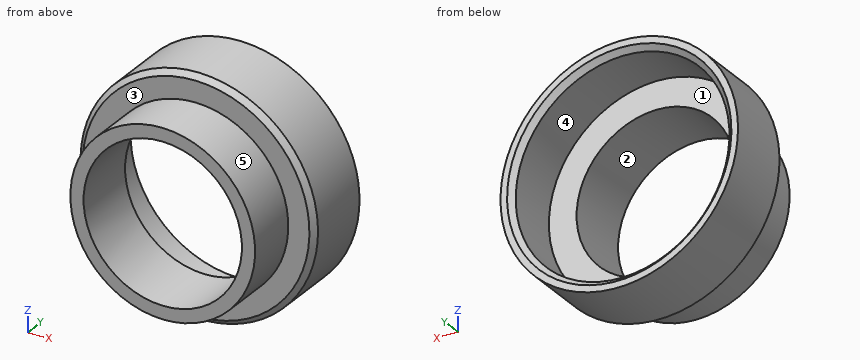
from build123d import *

# Parameters (mm, degrees)
SCHIZZO1_R        = 35
SCHIZZO1_R_2      = 30
ESTRUSIONE1_DEPTH = 30
ESTRUSIONE2_START = -10
SCHIZZO2_R        = 45
SCHIZZO2_R_2      = 30
ESTRUSIONE2_DEPTH = 5
SCHIZZO3_R        = 45
SCHIZZO3_R_2      = 40.5
ESTRUSIONE3_DEPTH = 22
SMUSSO1_SIZE      = 2
SMUSSO2_SIZE      = 2
SCHIZZO4_R        = 40.5
ESTRUSIONE4_DEPTH = 20


with BuildPart() as part:
    # Schizzo1 → Estrusione1 (new body)
    with BuildSketch(Plane(origin=(0, 0, 0), x_dir=(1, 0, 0), z_dir=(0, 1, 0))):
        with Locations(Location((0, 0, 0), (0, 0, 270))):
            Circle(SCHIZZO1_R)
        with Locations(Location((0, 0, 0), (0, 0, 270))):
            Circle(SCHIZZO1_R_2, mode=Mode.SUBTRACT)
    extrude(amount=ESTRUSIONE1_DEPTH)

    # Schizzo2 → Estrusione2 (add)
    with BuildSketch(Plane(origin=(0, 30, 0), x_dir=(1, 0, 0), z_dir=(0, 1, 0)).offset(ESTRUSIONE2_START)):
        with Locations(Location((0, 0, 0), (0, 0, 270))):
            Circle(SCHIZZO2_R)
        with Locations(Location((0, 0, 0), (0, 0, 270))):
            Circle(SCHIZZO2_R_2, mode=Mode.SUBTRACT)
    extrude(amount=ESTRUSIONE2_DEPTH)

    # Schizzo3 → Estrusione3 (add)
    with BuildSketch(Plane(origin=(0, 25, 0), x_dir=(1, 0, 0), z_dir=(0, 1, 0))):
        with Locations(Location((0, 0, 0), (0, 0, 270))):
            Circle(SCHIZZO3_R)
        with Locations(Location((0, 0, 0), (0, 0, 270))):
            Circle(SCHIZZO3_R_2, mode=Mode.SUBTRACT)
    extrude(amount=ESTRUSIONE3_DEPTH)

    # Smusso1
    smusso1_edges = [part.edges().sort_by_distance(p)[0] for p in [
        (0, 20, -45),
    ]]
    chamfer(smusso1_edges, length=SMUSSO1_SIZE)

    # Smusso2
    smusso2_edges = [part.edges().sort_by_distance(p)[0] for p in [
        (0, 47, -40.5),
    ]]
    chamfer(smusso2_edges, length=SMUSSO2_SIZE)

    # Schizzo4 → Estrusione4 (cut)
    with BuildSketch(Plane(origin=(0, 25, 0), x_dir=(1, 0, 0), z_dir=(0, 1, 0))):
        with Locations(Location((0, 0, 0), (0, 0, 270))):
            Circle(SCHIZZO4_R)
    extrude(amount=ESTRUSIONE4_DEPTH, mode=Mode.SUBTRACT)


solid = part.part
Build history of the part. All positions in model axes, mm. Face numbers are marked on the shaded views. A direction names the side the tool comes from. Give positions to 0.01 mm unless a question says otherwise; leave off trailing zeros. Order: outer loops, then holes, each group sorted by start corner. A loop starts at its lowest first (then second) coordinate and runs counter-clockwise, first axis right, second up. Notation, with made-up numbers: M -15,-15 L 25,-15 A14 ccw 25,3 Z; hole C -26,0.25 d6. An arc over 180 degrees is marked long. Use one line per item in the form item = value.
1) Probe probe 1 along Z at (x, y) = (0, 8); probe 2 along X at (y, z) = (32, 0). List the from-to ranges inside material, lowest first.
Calculated:
probe_1 = -35 to -30, 30 to 35
probe_2 = -45 to -40.5, 40.5 to 45
2) Tool access for the marked faces 1 and 2: list every direction of +Z, -Z, +X, -X, +Y, -Y with a clear straight run to the whole face (end or side of a thin tool).
Calculated:
face_1 = +Y
face_2 = +Y, -Y
3) Two-plate mould, pull along Z, no slides. Class the marked faces 3, 4 and 5: released by +Z, released by -Z, zero draft, split by the parting line, or undercut.
Calculated:
face_3 = zero draft
face_4 = undercut
face_5 = split by the parting line
4) Drop flat-ended pins along their axis: pin 1 (3 mm diameter, centred on y = 11, z = -13, fed in from -X); pin 2 (8 mm diameter, centred on y = 19.5, z = -31.5, fed in from -X); pin 3 (1 mm diameter, centred on x = -27.5, y = 31, fed in from -Z). Give the stop position or say it passes through.
Calculated:
pin_1 = -33.06
pin_2 = -34.92
pin_3 = -36
5) Saw through at C-C (y = 8). Give the cut face in (x, z).
Calculated:
outline = C 0,0 d70; hole C 0,0 d60
6) Saw through at A-A (x = 0). Give the cut face in (y, z).
Calculated:
outline = M 0,-35 L 20,-35 L 20,-43 L 22,-45 L 47,-45 L 47,-42.5 L 45,-40.5 L 25,-40.5 L 25,-30 L 0,-30 Z; M 0,30 L 25,30 L 25,40.5 L 45,40.5 L 47,42.5 L 47,45 L 22,45 L 20,43 L 20,35 L 0,35 Z
7) Saw through at B-B (z = 0). Give the cut face in (x, y).
Calculated:
outline = M -45,22 L -43,20 L -35,20 L -35,0 L -30,0 L -30,25 L -40.5,25 L -40.5,45 L -42.5,47 L -45,47 Z; M 30,0 L 35,0 L 35,20 L 43,20 L 45,22 L 45,47 L 42.5,47 L 40.5,45 L 40.5,25 L 30,25 Z
